Work out the finished part from the listing and answer in its coordinate system (mm). A direction names the side the tool comes from. Give positions to 0.01 mm unless a question says otherwise; leave off trailing zeros. Write each loop counter-clockwise with the first axis right and the second up, starting at its lowest first coordinate (ties: lowest second). Pieces come first, ordered by that corner, then holes.
1) Straight lines are drawn through the part: probe 1 along Z at (x, y) = (3.5, -2); probe 2 along X at (y, z) = (-1.95, -58.5); probe 3 along Y at (x, z) = (9.5, -8.5). For each, find the intervals that lie inside material, in ascending order.
2) A tool of negligible diameter and unlimited length cuts with its end or side. For faces 1 (the face through (17.912, -2.296, -11.593)), 2 (the face through (19.05, -2, -19)), 3 (the face through (10.389, -2, -57)), from which of +Z, -Z, +X, -X, +Y, -Y can it reach the whole face along a straight path? Write none if from no direction.
3) Find section A-A (x = 13.5). Determine the outline of the cut face in (y, z), plus the area to 3 significant figures.
4) Determine the mould class of faces 4 (the face through (10, -2.984, -31)), 5 (the face through (1.99, -1.15, -15.35)), 6 (the face through (1, -2, -39.688)) for opening direction Y: pulls with the +Y half, pulls with the -Y half, needs draft (parallel to the pull), parting line crosses it, or undercut.
5) Given pin 1 Ø1.8 at (x, y) = (0.5, 0) entering from -Z; pin 2 Ø0.7 at (y, z) = (-2, -18.5) entering from -X; pin 3 Ø0.7 at (x, y) = (12.5, -2) entering from +Z; pin 4 Ø3 at (x, y) = (0.5, -1) entering from -Z, each flat-ended and moving along its own axis, determine where each tip first touches the part or whether it passes through.
6) Find section B-B (y = 0.8). Determine the outline of the cut face in (x, z).
7) Find section D-D (x = -1). Determine the outline of the cut face in (y, z), plus the area to 3 significant figures.
8) Find section C-C (z = -46). Determine the outline of the cut face in (x, y), plus the area to 3 significant figures.
Autodesk Inventor part; units mm, degrees
ref_plane "YZ Plane" through (0, 0, 0) normal (1, 0, 0) x (0, 1, 0)
ref_plane "XZ Plane" through (0, 0, 0) normal (0, 1, 0) x (-1, 0, 0)
ref_plane "XY Plane" through (0, 0, 0) normal (0, 0, 1) x (1, 0, 0)
sketch "Sketch1" plane through (0, 0, 0) normal (0, 0, 1) x (1, 0, 0)
  line L0 (2.5847, -1.4923) -> (1.3748, -0.7938)
  arc A0 (2.5847, -1.4923) -> (0, -2.9845) centre (0, 0) ccw
  arc A1 (1.3748, -0.7938) -> (0, -1.5875) centre (0, 0) ccw
  arc A2 (1.3748, -0.7938) -> (0, -1.5875) centre (0, 0) ccw
  line L1 (0, -1.5875) -> (16.8049, -1.5875)
  line L2 (16.8049, -2.9845) -> (0, -2.9845)
  arc A3 (2.5847, -1.4923) -> (0, -2.9845) centre (0, 0) ccw
  line L3 (2.5847, -1.4923) -> (1.3748, -0.7938)
  line L4 (19.05, -1.5875) -> (16.8049, -1.5875)
  line L5 (19.05, -2.9845) -> (16.8049, -2.9845)
  line L6 (19.05, -1.5875) -> (19.05, -2.9845)
  point P0 (0, 0)
  point P1 (15.875, -2.9845)
extrude "Extrusion1" add sketch "Sketch1" against normal blind 63.5
sketch "Sketch2" plane through (0, -2.9845, 0) normal (0, -1, 0) x (1, 0, 0)
  line L0 (19.05, -23.1549) -> (19.05, -14.9451)
  line L1 (19.05, -14.9451) -> (16.8049, -12.7)
  line L2 (16.8049, -12.7) -> (19.05, -10.4549)
  line L3 (19.05, -10.4549) -> (19.05, -2.2451)
  line L4 (19.05, -2.2451) -> (16.8049, 0)
  line L5 (-2.9845, 0) -> (16.8049, 0)
  line L6 (0, -7.1247) -> (0, 0)
  line L7 (5.8525, -7.1247) -> (-2.9845, -7.1247)
  line L8 (5.8525, -39.6875) -> (5.8525, 0)
  line L9 (5.8525, -23.8125) -> (-2.9845, -23.8125)
  line L10 (0, -39.6875) -> (0, -23.8125)
  line L11 (5.8525, -39.6875) -> (-2.9845, -39.6875)
  line L12 (5.8525, -63.5) -> (5.8525, -39.6875)
  line L13 (-2.9845, -56.3753) -> (5.8525, -56.3753)
  line L14 (0, -63.5) -> (0, -56.3753)
  line L15 (16.8049, -63.5) -> (-2.9845, -63.5)
  line L16 (16.8049, -63.5) -> (19.05, -61.2549)
  line L17 (19.05, -61.2549) -> (19.05, -53.0451)
  line L18 (19.05, -53.0451) -> (16.8049, -50.8)
  line L19 (16.8049, -50.8) -> (19.05, -48.5549)
  line L20 (19.05, -48.5549) -> (19.05, -40.3451)
  line L21 (19.05, -40.3451) -> (16.8049, -38.1)
  line L22 (16.8049, -38.1) -> (19.05, -35.8549)
  line L23 (19.05, -35.8549) -> (19.05, -27.6451)
  line L24 (19.05, -27.6451) -> (16.8049, -25.4)
  line L25 (16.8049, -25.4) -> (19.05, -23.1549)
  line L26 (15.0114, -42.1386) -> (15.0114, -46.7614)
  line L27 (15.0114, -46.7614) -> (10.3886, -46.7614)
  line L28 (10.3886, -46.7614) -> (10.3886, -42.1386)
  line L29 (10.3886, -42.1386) -> (15.0114, -42.1386)
  line L30 (15.0114, -29.4386) -> (15.0114, -34.0614)
  line L31 (15.0114, -34.0614) -> (10.3886, -34.0614)
  line L32 (10.3886, -34.0614) -> (10.3886, -29.4386)
  line L33 (10.3886, -29.4386) -> (15.0114, -29.4386)
  line L34 (15.0114, -16.7386) -> (15.0114, -21.3614)
  line L35 (15.0114, -21.3614) -> (10.3886, -21.3614)
  line L36 (10.3886, -21.3614) -> (10.3886, -16.7386)
  line L37 (10.3886, -16.7386) -> (15.0114, -16.7386)
  line L38 (15.0114, -4.0386) -> (15.0114, -8.6614)
  line L39 (15.0114, -8.6614) -> (10.3886, -8.6614)
  line L40 (10.3886, -8.6614) -> (10.3886, -4.0386)
  line L41 (10.3886, -4.0386) -> (15.0114, -4.0386)
  line L42 (15.0114, -54.8386) -> (15.0114, -59.4614)
  line L43 (15.0114, -59.4614) -> (10.3886, -59.4614)
  line L44 (10.3886, -59.4614) -> (10.3886, -54.8386)
  line L45 (10.3886, -54.8386) -> (15.0114, -54.8386)
  line L46 (-2.9845, 0) -> (-2.9845, -63.5)
  line L47 (19.05, -53.0451) -> (19.05, -48.5549)
  line L48 (19.05, -40.3451) -> (19.05, -35.8549)
  line L49 (19.05, -27.6451) -> (19.05, -23.1549)
  line L50 (19.05, -14.9451) -> (19.05, -10.4549)
  line L51 (0, 0) -> (16.8049, 0)
  line L52 (16.8049, -63.5) -> (19.05, -63.5)
  line L53 (19.05, -63.5) -> (19.05, -61.2549)
  line L54 (19.05, -2.2451) -> (19.05, 0)
  line L55 (19.05, 0) -> (16.8049, 0)
  line L56 (16.8049, -63.5) -> (19.05, -61.2549)
  line L57 (19.05, -2.2451) -> (16.8049, 0)
  line L58 (0, -63.5) -> (16.8049, -63.5)
  line L59 (5.8525, -7.1247) -> (-2.9845, -7.1247)
  line L60 (-2.9845, -7.1247) -> (-2.9845, 0)
  line L61 (-2.9845, 0) -> (5.8525, 0)
  line L62 (5.8525, 0) -> (5.8525, -7.1247)
  point P0 (15.875, -31.75)
extrude "Extrusion2" cut sketch "Sketch2" against normal blind 6.35 contours L49 L24 L25 | L1 L2 L50 | L48 L21 L22 | L4 L55 L54 | L47 L18 L19 | L8 L7 L6 L5 | L6 L7 L46 L5 | L53 L52 L16 | L8 L11 L10 L9 | L10 L11 L46 L9 | L15 L14 L13 L12 | L15 L46 L13 L14 | L26 L27 L28 L29 | L30 L31 L32 L33 | L34 L35 L36 L37 | L38 L39 L40 L41 | L42 L43 L44 L45
sketch "Sketch3" plane through (0, -2.9845, 0) normal (0, -1, 0) x (1, 0, 0)
  line L0 (15.0114, -8.6614) -> (10.3886, -8.6614)
  circle A0 centre (12.7, -6.35) radius 2.3114
surface extrude "ExtrusionSrf1" sketch "Sketch3" against normal up to surface (1.397 mm away) shown no curves A0
pattern_linear "Rectangular Pattern1" count 5 spacing 12.7 along (0, 0, -1) of "ExtrusionSrf1"
properties part number "275-1272"
Results:
1. probe 1: z = -56.38 to -39.69, -23.81 to -7.12
1. probe 2: x = 5.85 to 10.39, 15.01 to 19.05
1. probe 3: y = -2.98 to -1.59
2. face 1: +X, +Y, -Y
2. face 2: +Z, -Z, +X, +Y, -Y
2. face 3: +Y, -Y
3. outline: (-2.98, -63.5) - (-1.59, -63.5) - (-1.59, -59.46) - (-2.98, -59.46) - close; (-2.98, -54.84) - (-1.59, -54.84) - (-1.59, -46.76) - (-2.98, -46.76) - close; (-2.98, -42.14) - (-1.59, -42.14) - (-1.59, -34.06) - (-2.98, -34.06) - close; (-2.98, -29.44) - (-1.59, -29.44) - (-1.59, -21.36) - (-2.98, -21.36) - close; (-2.98, -16.74) - (-1.59, -16.74) - (-1.59, -8.66) - (-2.98, -8.66) - close; (-2.98, -4.04) - (-1.59, -4.04) - (-1.59, 0) - (-2.98, 0) - close
3. area: 56.4 mm2
4. face 4: pulls with the -Y half
4. face 5: undercut
4. face 6: needs draft
5. pin 1: passes through
5. pin 2: stops at x = -2.49
5. pin 3: stops at z = 0
5. pin 4: stops at z = -56.38
6. outline: (-2.88, -56.38) - (-1.37, -56.38) - (-1.37, -39.69) - (-2.88, -39.69) - close; (-2.88, -23.81) - (-1.37, -23.81) - (-1.37, -7.12) - (-2.88, -7.12) - close; (1.37, -56.38) - (2.88, -56.38) - (2.88, -39.69) - (1.37, -39.69) - close; (1.37, -23.81) - (2.88, -23.81) - (2.88, -7.12) - (1.37, -7.12) - close
7. outline: (-2.81, -56.38) - (-1.23, -56.38) - (-1.23, -39.69) - (-2.81, -39.69) - close; (-2.81, -23.81) - (-1.23, -23.81) - (-1.23, -7.12) - (-2.81, -7.12) - close; (1.23, -56.38) - (2.81, -56.38) - (2.81, -39.69) - (1.23, -39.69) - close; (1.23, -23.81) - (2.81, -23.81) - (2.81, -7.12) - (1.23, -7.12) - close
7. area: 105 mm2
8. outline: (0, -2.98) - (10.39, -2.98) - (10.39, -1.59) - (0, -1.59) arc R1.59 cw (long way) to (1.37, -0.79) - (2.58, -1.49) arc R2.98 ccw (long way) to start; (15.01, -2.98) - (19.05, -2.98) - (19.05, -1.59) - (15.01, -1.59) - close
8. area: 36.9 mm2
